Part model, mm, in its own coordinate system. A direction names the side the tool comes from. Give positions to 0.01 mm unless a question says otherwise; leave off trailing zeros. Order: outer loops, then holes, each group sorted by start corner. A loop starts at its lowest first (then second) coordinate and runs counter-clockwise, first axis right, second up.
from build123d import *

# Parameters (mm, degrees)
SKETCH1_W           = 46.4
SKETCH1_H           = 24.75
BOSS_EXTRUDE1_DEPTH = 5.9
BOSS_EXTRUDE2_DEPTH = 2.5
SKETCH3_W           = 50
SKETCH3_H           = 50
BOSS_EXTRUDE3_DEPTH = 2.5
SKETCH4_W           = 46.4
SKETCH4_H           = 0.93
BOSS_EXTRUDE4_DEPTH = 5.9
SKETCH5_W           = 46.4
SKETCH5_H           = 0.93
BOSS_EXTRUDE5_DEPTH = 5.9
SKETCH6_W           = 46.4
SKETCH6_H           = 3
BOSS_EXTRUDE6_DEPTH = 8.4
SKETCH7_W           = 46.4
SKETCH7_H           = 3
BOSS_EXTRUDE7_DEPTH = 8.4


with BuildPart() as part:
    # Sketch1 → Boss-Extrude1 (new body)
    with BuildSketch(Plane(origin=(0, 0, 0), x_dir=(1, 0, 0), z_dir=(0, 1, 0))):
        Rectangle(SKETCH1_W, SKETCH1_H)
    extrude(amount=BOSS_EXTRUDE1_DEPTH)

    # Sketch2 → Boss-Extrude2 (add)
    with BuildSketch(Plane(origin=(0, 5.9, 0), x_dir=(1, 0, 0), z_dir=(0, 1, 0))):
        Polygon((23.2, -11.45), (23.2, 0), (23.2, 11.45), (-23.2, 11.45), (-23.2, -11.45), align=None)
    extrude(amount=BOSS_EXTRUDE2_DEPTH)

    # Sketch3 → Boss-Extrude3 (add)
    with BuildSketch(Plane.XZ):
        Rectangle(SKETCH3_W, SKETCH3_H)
    extrude(amount=BOSS_EXTRUDE3_DEPTH)

    # Sketch4 → Boss-Extrude4 (add)
    with BuildSketch(Plane(origin=(0, 0, 0), x_dir=(1, 0, 0), z_dir=(0, 1, 0))):
        with Locations((0, 13.64)):
            Rectangle(SKETCH4_W, SKETCH4_H)
    extrude(amount=BOSS_EXTRUDE4_DEPTH)

    # Sketch5 → Boss-Extrude5 (add)
    with BuildSketch(Plane(origin=(0, 0, 0), x_dir=(1, 0, 0), z_dir=(0, 1, 0))):
        with Locations((0, -13.64)):
            Rectangle(SKETCH5_W, SKETCH5_H)
    extrude(amount=BOSS_EXTRUDE5_DEPTH)

    # Sketch6 → Boss-Extrude6 (add)
    with BuildSketch(Plane(origin=(0, 0, 0), x_dir=(1, 0, 0), z_dir=(0, 1, 0))):
        with Locations((0, 15.605)):
            Rectangle(SKETCH6_W, SKETCH6_H)
    extrude(amount=BOSS_EXTRUDE6_DEPTH)

    # Sketch7 → Boss-Extrude7 (add)
    with BuildSketch(Plane(origin=(0, 0, 0), x_dir=(1, 0, 0), z_dir=(0, 1, 0))):
        with Locations((0, -15.605)):
            Rectangle(SKETCH7_W, SKETCH7_H)
    extrude(amount=BOSS_EXTRUDE7_DEPTH)


solid = part.part
Item 1: Band-saw the part on D-D on y = 7.5. List the corners of the cut face in (x, z) (3 decimals).
Item 2: Band-saw the part on A-A on y = 2.5. List the corners of the cut face in (x, z) (3 decimals).
Item 3: Which spindle directions (+Z, -Z, +X, -X, +Y, -Y) get a long thin tool onto all of the face, cutting with end or side? Do faces 1 (the face through (0, 7, -14.105)), 2 (the face through (-23.2, 4, 15)), 3 (the face through (23.2, 4, 0)). Say none if no direction does.
Item 4: Band-saw the part on C-C on x = -20.5. List the corners of the cut face in (y, z) (3 decimals).
Item 5: Drop flat-ended pins along their axis: P1, Ø1, axis at x = 6.5, z = -13.5, coming from the +Y side; P2, Ø2, axis at y = 2.5, z = 15.5, coming from the -X side; P3, Ø3, axis at x = 7.5, y = 7, coming from the -Z side (3 decimals); P4, Ø6.5, axis at x = -10.5, y = 2, coming from the -Z side. Give the stop position or say it passes through.
Item 6: Pull direction Z, two halves, no side cores. Call faces 4 (the face through (0, 4, 17.105)), 5 (the face through (0, 3, 13.175)), 6 (the face through (0, 7, 14.105)), 7 (the face through (-23.2, 4, -15)): released by +Z, released by -Z, zero draft, split by the parting line, or undercut.
Item 7: Drill centre lines: probe 1 along Z at (x, y) = (1.5, 2.5) (3 decimals); probe 2 along Z at (x, y) = (0, 6.25) (3 decimals); probe 3 along X at (y, z) = (6.5, -2). Where is each one in solid material? Low to high.
Item 8: Band-saw the part on B-B on z = -15.5. List the corners of the cut face in (x, y), plus the area to 3 significant figures.
Working result:
1. outline: (-23.2, -17.105) - (23.2, -17.105) - (23.2, -14.105) - (-23.2, -14.105) - close; (-23.2, -11.45) - (23.2, -11.45) - (23.2, 11.45) - (-23.2, 11.45) - close; (-23.2, 14.105) - (23.2, 14.105) - (23.2, 17.105) - (-23.2, 17.105) - close
2. outline: (-23.2, -17.105) - (23.2, -17.105) - (23.2, -13.175) - (-23.2, -13.175) - close; (-23.2, -12.375) - (23.2, -12.375) - (23.2, 12.375) - (-23.2, 12.375) - close; (-23.2, 13.175) - (23.2, 13.175) - (23.2, 17.105) - (-23.2, 17.105) - close
3. face 1: +X, -X, +Y
3. face 2: +Z, -Z, -X, +Y
3. face 3: +Z, -Z, +X, +Y
4. outline: (-2.5, -25) - (0, -25) - (0, -17.105) - (8.4, -17.105) - (8.4, -14.105) - (5.9, -14.105) - (5.9, -13.175) - (0, -13.175) - (0, -12.375) - (5.9, -12.375) - (5.9, -11.45) - (8.4, -11.45) - (8.4, 11.45) - (5.9, 11.45) - (5.9, 12.375) - (0, 12.375) - (0, 13.175) - (5.9, 13.175) - (5.9, 14.105) - (8.4, 14.105) - (8.4, 17.105) - (0, 17.105) - (0, 25) - (-2.5, 25) - close
5. P1: stops at y = 5.9
5. P2: stops at x = -23.2
5. P3: stops at z = -17.105
5. P4: stops at z = -25
6. face 4: released by +Z
6. face 5: undercut
6. face 6: undercut
6. face 7: zero draft
7. probe 1: z = -17.105 to -13.175, -12.375 to 12.375, 13.175 to 17.105
7. probe 2: z = -17.105 to -14.105, -11.45 to 11.45, 14.105 to 17.105
7. probe 3: x = -23.2 to 23.2
8. outline: (-25, -2.5) - (25, -2.5) - (25, 0) - (23.2, 0) - (23.2, 8.4) - (-23.2, 8.4) - (-23.2, 0) - (-25, 0) - close
8. area: 515 mm2
